Model file for the job. Use its own axes, mm. Face numbers are marked on the shaded views. A direction names the side the tool comes from. Round coordinates to 2 decimals unless told otherwise and drop trailing zeros. Write each loop counter-clockwise with the first axis right and the second up, starting at its lowest first coordinate (ties: lowest second). Pieces come first, ordered by that corner, then holes. Notation, with made-up numbers: (89.25, 35.25) - (135.25, 35.25) arc R25 cw to (135.25, 54.25) - close; hole circle Ø9 at (40, 83). An arc over 180 degrees is marked (long way). One line per item, written item: value.
from build123d import *

# Parameters (mm, degrees)
ESQUISSE1_R             = 5
ESQUISSE1_R_2           = 2.75
BOSS_EXTRU_1_DEPTH      = 3
BOSS_EXTRU_2_DEPTH      = 1
BOSS_EXTRU_2_DEPTH_BACK = 1
CONG_1_R                = 1


with BuildPart() as part:
    # Esquisse1 → Boss.-Extru.1 (new body)
    with BuildSketch(Plane.XY):
        Circle(ESQUISSE1_R)
        Circle(ESQUISSE1_R_2, mode=Mode.SUBTRACT)
    extrude(amount=BOSS_EXTRU_1_DEPTH)

    # Esquisse2 → Boss.-Extru.2 (add, two sides: drawn at the far end of the back side and taken through both)
    with BuildSketch(Plane(origin=(0, 0, 0), x_dir=(1, 0, 0), z_dir=(0, 1, 0)).offset(-BOSS_EXTRU_2_DEPTH_BACK)):
        with BuildLine():
            Line((-5, 0), (-11.278292154, -4.43596899))
            ThreePointArc((-11.278292154, -4.43596899), (-12.095263684, -5.73045857), (-11.757607433, -7.223487038))
            Line((-11.757607433, -7.223487038), (-11.382926754, -7.753778113))
            ThreePointArc((-11.382926754, -7.753778113), (-9.972806189, -8.587172352), (-8.41291055, -8.087460876))
            Line((-8.41291055, -8.087460876), (-2.75, -3))
            Line((-2.75, -3), (-5, 0))
        make_face()
        with BuildLine():
            Line((8.41291055, -8.087460876), (2.75, -3))
            Line((2.75, -3), (5, 0))
            Line((5, 0), (11.278292154, -4.43596899))
            ThreePointArc((11.278292154, -4.43596899), (12.095263684, -5.73045857), (11.757607433, -7.223487038))
            Line((11.757607433, -7.223487038), (11.382926754, -7.753778113))
            ThreePointArc((11.382926754, -7.753778113), (9.972806189, -8.587172352), (8.41291055, -8.087460876))
        make_face()
    extrude(amount=BOSS_EXTRU_2_DEPTH + BOSS_EXTRU_2_DEPTH_BACK)

    # Congé1
    cong_1_edges = [part.edges().sort_by_distance(p)[0] for p in [
        (0, 5, 3),
        (0, -5, 3),
    ]]
    fillet(cong_1_edges, radius=CONG_1_R)


solid = part.part
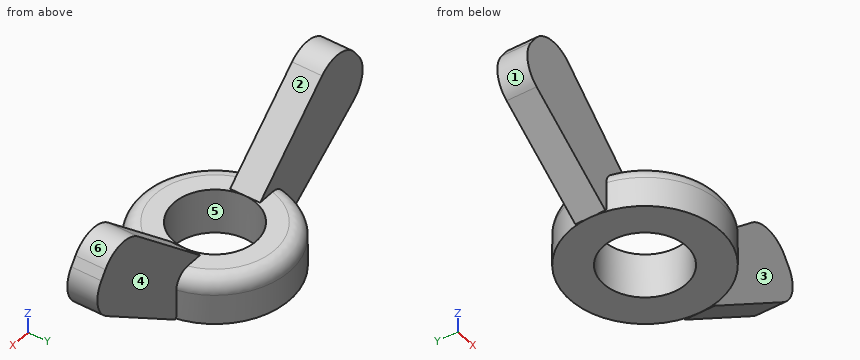
1. Band-saw the part on A-A on x = 0. Write the cut outline in (y, z).
Report:
outline: (-5, 0) - (-2.75, 0) - (-2.75, 3) - (-4, 3) arc R1 ccw to (-5, 2) - close; (2.75, 0) - (5, 0) - (5, 2) arc R1 ccw to (4, 3) - (2.75, 3) - close
2. Band-saw the part on B-B on z = 6. Write the cut outline in (x, y).
Report:
outline: (-12.12, -1) - (-6.09, -1) - (-6.09, 1) - (-12.12, 1) - close; (6.09, -1) - (12.12, -1) - (12.12, 1) - (6.09, 1) - close
3. Mould opens along Y. For the marked faces 3, 4, 5 and 6 say: released by +Y, released by -Y, zero draft, split by the parting line, or undercut.
Report:
face 3: released by -Y
face 4: released by +Y
face 5: undercut
face 6: zero draft
4. Wall check: probe 1 along Z at (x, y) = (3, -2); probe 2 along Y at (x, z) = (-1, 2.75); probe 3 along X at (y, z) = (1.75, 1). Give the ranges that are in metal, low to high. Write a range as [from, to].
Report:
probe 1: [0, 3]
probe 2: [-4.55, -2.56], [2.56, 4.55]
probe 3: [-4.68, -2.12], [2.12, 4.68]
5. Band-saw the part on D-D on z = 1. Write the cut outline in (x, y), plus the area to 3 significant figures.
Report:
outline: (-6.42, -1) - (-4.9, -1) arc R5 ccw to (4.9, -1) - (6.42, -1) - (6.42, 1) - (4.9, 1) arc R5 ccw to (-4.9, 1) - (-6.42, 1) - close; hole circle Ø5.5 at (0, 0)
area: 60.6 mm²
6. Tool access for the marked faces 1 and 2: list every direction of +Z, -Z, +X, -X, +Y, -Y with a clear straight run to the whole face (end or side of a thin tool).
Report:
face 1: -X, +Y, -Y
face 2: +Z, +Y, -Y
7. Drop flat-ended pins along their axis: pin 1 (3 mm diameter, centred on x = -1, y = -2, fed in from +Z); pin 2 (4 mm diameter, centred on x = 4, y = 3, fed in from -Z); pin 3 (2 mm diameter, centred on y = -1, z = 3, fed in from -X); pin 4 (4 mm diameter, centred on x = -5.5, y = -1, fed in from +Z). Give the stop position or say it passes through.
Report:
pin 1: z = 3
pin 2: z = 0
pin 3: x = -10.66
pin 4: z = 7.27
